Autodesk Inventor part; units mm, degrees
ref_plane "YZ Plane" through (0, 0, 0) normal (1, 0, 0) x (0, 1, 0)
ref_plane "XZ Plane" through (0, 0, 0) normal (0, 1, 0) x (-1, 0, 0)
ref_plane "XY Plane" through (0, 0, 0) normal (0, 0, 1) x (1, 0, 0)
sketch "Sketch1" plane through (0, 0, 0) normal (0, 1, 0) x (-1, 0, 0)
  line L0 (15, 6) -> (-15, 6)
  line L1 (-15, 6) -> (-15, 0)
  line L2 (-15, 0) -> (15, 0)
  line L3 (15, 0) -> (15, 6)
  point P0 (0, 0)
  dimension "d0" = 30
extrude "Extrusion1" add sketch "Sketch1" along normal blind 10
sketch "Sketch2" plane through (-15, 0, 6) normal (0, 0, 1) x (1, 0, 0)
  circle A0 centre (15, 0) radius 6
  line L0 (30, 10) -> (0, 10)
  line L1 (30, 10) -> (24, 10)
  line L2 (24, 10) -> (24, 4)
  line L3 (24, 4) -> (30, 4)
  line L4 (30, 4) -> (30, 10)
  line L5 (0, 0) -> (0, 10)
  line L6 (0, 10) -> (6, 10)
  line L7 (6, 10) -> (6, 4)
  line L8 (6, 4) -> (0, 4)
  line L9 (0, 4) -> (0, 10)
  arc A1 (24, 4) -> (6, 4) centre (15, -0.5678) ccw
  line L10 (6, 10) -> (24, 10)
  dimension "d3" = 12
  dimension "d4" = 6
  dimension "d5" = 6
  dimension "d6" = 6
extrude "Extrusion2" cut sketch "Sketch2" against normal blind 10
sketch "Sketch3" plane through (0, 0, 0) normal (0, -1, 0) x (1, 0, 0)
  circle A0 centre (-12, 3) radius 2
  circle A1 centre (12, 3) radius 2
  point P0 (0, 0)
  dimension "d9" = 4
  dimension "d10" = 4
extrude "Extrusion3" cut sketch "Sketch3" against normal blind 10
properties part number "printHeadMount"
The listing builds one solid part. Answer for the finished solid, in the listing's coordinates (mm). A direction names the side the tool comes from. Give positions to 0.01 mm unless a question says otherwise; leave off trailing zeros. Loops run counter-clockwise (first coordinate to the right, second up) from the corner with the lowest first, then second, coordinate; pieces in that order, holes last. Notation, with made-up numbers: M 75,11.25 L 122,11.25 A24 ccw 122,25.25 Z; hole C 45.5,87 d7. An arc over 180 degrees is marked long. One line per item, written item: value.
1. For a pull along X with two mould halves and no side action, classify faces 4 (the face through (9.6, 0, 3)), 5 (the face through (-15, 2, 3)), 6 (the face through (0, 6, 3)) as pulls with the +X half, pulls with the -X half, needs draft (parallel to the pull), parting line crosses it, or undercut.
Found:
face 4: needs draft
face 5: pulls with the -X half
face 6: undercut
2. Section A-A on x = 12 is taken. Determine the outline of the cut face in (y, z).
Found:
outline: M 0,0 L 4,0 L 4,1 L 0,1 Z; M 0,5 L 4,5 L 4,6 L 0,6 Z
3. Section C-C on z = 5.3 is taken. Determine the outline of the cut face in (x, y), plus the area to 3 significant figures.
Found:
outline: M -15,0 L -6,0 A6 cw 6,0 L 15,0 L 15,4 L 9,4 A10.09 ccw -9,4 L -15,4 Z
area: 135 mm^2
4. Find the intervals of material crossed by probe 1 along Z at (x, y) = (12, 2.8); probe 2 along X at (y, z) = (2.25, 4); probe 3 along X at (y, z) = (4.5, 3.75), in increasing order.
Found:
probe 1: 0 to 1, 5 to 6
probe 2: -15 to -13.73, -10.27 to -5.56, 5.56 to 10.27, 13.73 to 15
probe 3: -8.73 to -3.97, 3.97 to 8.73
5. Section B-B on z = 3 is taken. Determine the outline of the cut face in (x, y).
Found:
outline: M -15,0 L -14,0 L -14,4 L -15,4 Z; M -10,0 L -6,0 A6 cw 6,0 L 10,0 L 10,4 L 9,4 A10.09 ccw -9,4 L -10,4 Z; M 14,0 L 15,0 L 15,4 L 14,4 Z
6. For faces 1 (the face through (0, 7, 0)), 2 (the face through (11, 4, 5)), 3 (the face through (-11, 4, 5)), determine the directions among +Z, -Z, +X, -X, +Y, -Y from which every point of the face is accessible in a straight line to the end or side of a thin tool.
Found:
face 1: -Z, +X, -X, +Y, -Y
face 2: +Z, -Z, +X, +Y
face 3: +Z, -Z, -X, +Y
7. Section D-D on y = 3.25 is taken. Determine the outline of the cut face in (x, z).
Found:
outline: M -15,0 L -5.04,0 L -5.04,6 L -15,6 Z; M 5.04,0 L 15,0 L 15,6 L 5.04,6 Z; hole C -12,3 d4; hole C 12,3 d4
8. Each of these flat-tipped pins is pushed along its axis until it touches: P1, Ø3, axis at x = -13, z = 2, coming from the +Y side; P2, Ø1.5, axis at y = 6, z = 1, coming from the -X side. Where does it stop, or does it pass through?
Found:
P1: y = 4
P2: x = -8.25
